For this review, take the finished solid that the model builds, in its own axes (mm). Round coordinates to 2 decimals unless told otherwise and drop trailing zeros. Write each loop counter-clockwise with the first axis right and the second up, starting at its lowest first coordinate (ties: lowest second). Pieces come first, ordered by that corner, then holes. Notation, with made-up numbers: (77.25, 67) -> (100.25, 67) arc R25 ccw to (100.25, 94) -> close; hole circle Ø11 at (-31.75, 51.25). An arc over 180 degrees is marked (long way). Answer in a Markdown table with one row per item.
from build123d import *

# Parameters (mm, degrees)
SKETCH_R   = 24
SKETCH_R_2 = 7
SKETCH_R_3 = 2.55
SKETCH_R_4 = 1.5
PAD_DEPTH  = 3


with BuildPart() as part:
    # Sketch → Pad (new body)
    with BuildSketch(Plane.XY):
        Polygon((-123, 33.25), (-115, 33.25), (-115, 36.25), (115, 36.25), (115, 33.25), (123, 33.25), (123, -33.25), (115, -33.25), (115, -36.25), (-115, -36.25), (-115, -33.25), (-123, -33.25), align=None)
        with Locations((0, 4.25)):
            Circle(SKETCH_R, mode=Mode.SUBTRACT)
        with Locations((-101, 4.25)):
            Circle(SKETCH_R_2, mode=Mode.SUBTRACT)
        with Locations((-73, 4.25)):
            Circle(SKETCH_R_2, mode=Mode.SUBTRACT)
        with Locations((73, 4.25)):
            Circle(SKETCH_R_2, mode=Mode.SUBTRACT)
        with Locations((101, 4.25)):
            Circle(SKETCH_R_2, mode=Mode.SUBTRACT)
        with Locations((-101, 19.25)):
            Circle(SKETCH_R_3, mode=Mode.SUBTRACT)
        with Locations((-73, 19.25)):
            Circle(SKETCH_R_3, mode=Mode.SUBTRACT)
        with Locations((73, 19.25)):
            Circle(SKETCH_R_3, mode=Mode.SUBTRACT)
        with Locations((101, 19.25)):
            Circle(SKETCH_R_3, mode=Mode.SUBTRACT)
        with Locations((-119, 30.45)):
            Circle(SKETCH_R_4, mode=Mode.SUBTRACT)
        with Locations((119, 30.45)):
            Circle(SKETCH_R_4, mode=Mode.SUBTRACT)
    extrude(amount=PAD_DEPTH)


solid = part.part
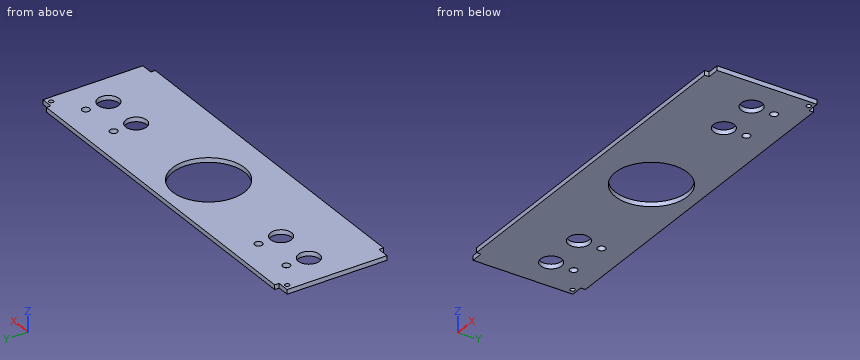
1) Consider section D-D on y = -5. State the section outline as (x, z) points, then the cut area to 3 significant figures.
Solved:
| item | result |
|---|---|
| outline | (-123, 0) -> (-22.15, 0) -> (-22.15, 3) -> (-123, 3) -> close; (22.15, 0) -> (123, 0) -> (123, 3) -> (22.15, 3) -> close |
| area | 605 mm² |
2) Consider section B-B on y = 4.25. State the section outline as (x, z) points.
Solved:
| item | result |
|---|---|
| outline | (-123, 0) -> (-108, 0) -> (-108, 3) -> (-123, 3) -> close; (-94, 0) -> (-80, 0) -> (-80, 3) -> (-94, 3) -> close; (-66, 0) -> (-24, 0) -> (-24, 3) -> (-66, 3) -> close; (24, 0) -> (66, 0) -> (66, 3) -> (24, 3) -> close; (80, 0) -> (94, 0) -> (94, 3) -> (80, 3) -> close; (108, 0) -> (123, 0) -> (123, 3) -> (108, 3) -> close |
3) Consider section A-A on x = 0. State the section outline as (y, z) points, then the cut area to 3 significant figures.
Solved:
| item | result |
|---|---|
| outline | (-36.25, 0) -> (-19.75, 0) -> (-19.75, 3) -> (-36.25, 3) -> close; (28.25, 0) -> (36.25, 0) -> (36.25, 3) -> (28.25, 3) -> close |
| area | 73.5 mm² |
4) For line 1 (Y direction, x = 101, z = 2.15); line 2 (Y direction, x = 0, z = 1.75); line 3 (Y direction, x = -119, z = 1.1), list the stretches that pass through material, from the lowest coordinate up. Write a range as [from, to].
Solved:
| item | result |
|---|---|
| line 1 | [-36.25, -2.75], [11.25, 16.7], [21.8, 36.25] |
| line 2 | [-36.25, -19.75], [28.25, 36.25] |
| line 3 | [-33.25, 28.95], [31.95, 33.25] |
5) Consider section C-C on x = 73. State the section outline as (y, z) points, then the cut area to 3 significant figures.
Solved:
| item | result |
|---|---|
| outline | (-36.25, 0) -> (-2.75, 0) -> (-2.75, 3) -> (-36.25, 3) -> close; (11.25, 0) -> (16.7, 0) -> (16.7, 3) -> (11.25, 3) -> close; (21.8, 0) -> (36.25, 0) -> (36.25, 3) -> (21.8, 3) -> close |
| area | 160 mm² |
6) Clearance check with flat-ended pins moving along their axes: pin 1 Ø0.9 at (x, z) = (-118.5, 2) entering from +Y; pin 2 Ø0.9 at (x, z) = (119.5, 2) entering from -Y; pin 3 Ø1.5 at (y, z) = (-34.5, 2) entering from +X. State where each tip first meets the part, or that it passes through.
Solved:
| item | result |
|---|---|
| pin 1 | y = 33.25 |
| pin 2 | y = -33.25 |
| pin 3 | x = 115 |
